from build123d import *

# Parameters (mm, degrees)
CUT_EXTRUDE1_DEPTH  = 320.36859803
SKETCH3_R           = 3.675
CUT_EXTRUDE2_DEPTH  = 320.36859803
SKETCH8_R           = 65.405
SKETCH8_R_2         = 52.705
BOSS_EXTRUDE1_DEPTH = 127
SKETCH9_R           = 63.5
SKETCH9_R_2         = 2.5
CUT_EXTRUDE4_DEPTH  = 127


# Read off the part's stored shape, not the designer's step: Shell1
with BuildPart() as part:
    # Sketch1 → Revolve1 (revolve)
    with BuildSketch(Plane(origin=(0, 0, 0), x_dir=(1, 0, 0), z_dir=(0, 1, 0))):
        with BuildLine():
            Line((0, 431.8), (0, 101.6))
            Line((0, 101.6), (65.405, 101.6))
            ThreePointArc((65.405, 101.6), (48.896438034, 269.907645418), (0, 431.8))
        make_face()
    revolve(axis=Axis((0, 0, -431.8), (0, 0, 1)))

    # Shell1 outline → Shell1 (revolve, cut)
    with BuildSketch(Plane.XZ):
        with BuildLine():
            add(Edge.make_bspline(
                [(59.055, -101.6), (59.055, -263.749938118), (0, -414.763544811)],
                knots=[0, 0, 0, 0.372773614, 0.372773614, 0.372773614], degree=2, weights=[1, 0.982680207, 1]))
            Line((59.055, -101.6), (0, -101.5999999))
            Line((0, -101.5999999), (0, -414.763544811))
        make_face()
    revolve(axis=Axis((0, 0, 0), (0, 0, 1)), mode=Mode.SUBTRACT)

    # Sketch2 → Cut-Extrude1 (cut, through all)
    with BuildSketch(Plane.XY.offset(-407.280672059)):
        Polygon((0, 6.076611583), (-5.2625, 3.038305792), (-5.2625, -3.038305792), (0, -6.076611583), (5.2625, -3.038305792), (5.2625, 3.038305792), align=None)
    extrude(amount=CUT_EXTRUDE1_DEPTH, mode=Mode.SUBTRACT)

    # Sketch3 → Cut-Extrude2 (cut, through all)
    with BuildSketch(Plane.XY.offset(-407.280672059)):
        Circle(SKETCH3_R)
    extrude(amount=-CUT_EXTRUDE2_DEPTH, mode=Mode.SUBTRACT)

    # Sketch8 → Boss-Extrude1 (add)
    with BuildSketch(Plane.XY.offset(-101.6)):
        Circle(SKETCH8_R)
        Circle(SKETCH8_R_2, mode=Mode.SUBTRACT)
    extrude(amount=BOSS_EXTRUDE1_DEPTH)

    # Sketch9 → Cut-Extrude4 (cut)
    with BuildSketch(Plane.XY.offset(25.4)):
        Circle(SKETCH9_R)
        Circle(SKETCH9_R_2, mode=Mode.SUBTRACT)
    extrude(amount=-CUT_EXTRUDE4_DEPTH, mode=Mode.SUBTRACT)


solid = part.part
Geometry check sheet. Reference: the model listing, model coordinates, mm. A direction names the side the tool comes from. Round coordinates to 2 decimals unless told otherwise and drop trailing zeros. Loops run counter-clockwise (first coordinate to the right, second up) from the corner with the lowest first, then second, coordinate; pieces in that order, holes last.
Item 1: Access from +Z, -Z, +X, -X, +Y, -Y to the whole of each face (thin tool, end or side, straight path). Record for faces 4 (the cylindrical face through (-13.77, -61.99, -37.21)), 5 (the cylindrical face through (-0.797, -3.588, -414.903)).
Item 2: Cross-section at A-A on z = -63. Record the boundary of the cut face in (x, y) (3 decimals), then the cut area to 3 significant figures.
Item 3: Thickness scan on line 1 (Y direction, x = 0, z = -23.5) (3 decimals); line 2 (X direction, y = -44.5, z = -24); line 3 (Y direction, x = 0, z = -418) (3 decimals). Record the ranges inside material, lowest first.
Item 4: Gauge pin test, flat ends, axial feed: pin 1 (5 mm diameter, centred on x = -8.5, z = -20.5, fed in from -Y); pin 2 (1.5 mm diameter, centred on y = 46, z = -90, fed in from -X); pin 3 (3 mm diameter, centred on y = -5.5, z = -229, fed in from -X). Record the tip position at first contact, or that the pin passes through.
Item 5: Mould release check, pull along X, two halves, no side actions. Record for faces 1 (the flat face through (-54, 34, 25.4)), 2 (the cylindrical face through (-14.18, -63.85, -38.99)), 3 (the flat face through (-4, -1, -407.281)): pulls with the +X half, pulls with the -X half, needs draft (parallel to the pull), parting line crosses it, or undercut.
Answer sheet:
1. face 4: +Z
1. face 5: +Z, -Z
2. outline: circle Ø130.81 at (0, 0); hole circle Ø127 at (0, 0)
2. area: 771 mm2
3. line 1: y = -65.405 to -63.5, 63.5 to 65.405
3. line 2: x = -47.93 to -45.3, 45.3 to 47.93
3. line 3: y = -5.552 to -3.675, 3.675 to 5.552
4. pin 1: stops at y = -65.13
4. pin 2: stops at x = -47.23
4. pin 3: stops at x = -55.98
5. face 1: needs draft
5. face 2: parting line crosses it
5. face 3: undercut
